Build history of the part. All positions in model axes, mm. A direction names the side the tool comes from. Round coordinates to 2 decimals unless told otherwise and drop trailing zeros. Order: outer loops, then holes, each group sorted by start corner. A loop starts at its lowest first (then second) coordinate and runs counter-clockwise, first axis right, second up. Notation, with made-up numbers: M 10.25,-13.75 L 17.25,-13.75 A27 cw 17.25,24.25 Z; hole C 54.25,-29.5 d9. An arc over 180 degrees is marked long. One line per item, written item: value. Start each with the question number.
Item 1: Tool access for faces 1 (the flat face through (0, 29, -3.099)), 2 (the flat face through (0, 0, 0)), 3 (the flat face through (0, 23.065, -4)): list every direction of +Z, -Z, +X, -X, +Y, -Y with a clear straight run to the whole face (end or side of a thin tool).
Item 2: Probe L1, parallel to Y at x = 4, z = -10; L2, parallel to Y at x = 1, z = -5.25 (3 decimals); L3, parallel to Z at x = -3.5, y = 24.5. List the from-to ranges inside material, lowest first.
Item 3: Band-saw the part on A-A, the plane z = 0. Write the cut outline in (x, y) (1 decimal).
Item 4: Band-saw the part on B-B, the plane x = 0. Write the cut outline in (y, z) (1 decimal), then the cut area to 3 significant figures.
Item 5: Band-saw the part on C-C, the plane y = 5.5. Write the cut outline in (x, z) (1 decimal).
Item 6: Band-saw the part on D-D, the plane y = 21.5. Write the cut outline in (x, z).
Item 7: Pin check, flat tips, straight feed: pin 1 (1 mm diameter, centred on y = 5.5, z = 8, fed in from +X); pin 2 (2 mm diameter, centred on x = 1, z = 4.5, fed in from -Y); pin 3 (5 mm diameter, centred on x = 6.5, y = 9, fed in from -Z); pin 4 (8 mm diameter, centred on y = 11.5, z = 6.5, fed in from +X). Stop position of each tip, or through.
```python
from build123d import *

# Parameters (mm, degrees)
SKETCH1_R           = 11.1125
BOSS_EXTRUDE1_DEPTH = 13.54
SKETCH2_R           = 5.5245
BOSS_EXTRUDE2_DEPTH = 9.525
BOSS_EXTRUDE3_DEPTH = 12.7


with BuildPart() as part:
    # Sketch1 → Boss-Extrude1 (new body)
    with BuildSketch(Plane(origin=(0, 0, 0), x_dir=(1, 0, 0), z_dir=(0, 1, 0))):
        with Locations(Location((0, 0, 0), (0, 0, 270))):
            Circle(SKETCH1_R)
    extrude(amount=BOSS_EXTRUDE1_DEPTH)

    # Sketch2 → Boss-Extrude2 (add)
    with BuildSketch(Plane(origin=(0, 13.54, 0), x_dir=(1, 0, 0), z_dir=(0, 1, 0))):
        with Locations(Location((0, 0, 0), (0, 0, 90))):
            Circle(SKETCH2_R)
    extrude(amount=BOSS_EXTRUDE2_DEPTH)

    # Sketch3 → Boss-Extrude3 (add)
    with BuildSketch(Plane(origin=(0, 23.065, 0), x_dir=(1, 0, 0), z_dir=(0, 1, 0))):
        with BuildLine():
            Line((2.387059513, 3.0988), (-2.387059513, 3.0988))
            ThreePointArc((-2.387059513, 3.0988), (0, -3.9116), (2.387059513, 3.0988))
        make_face()
    extrude(amount=BOSS_EXTRUDE3_DEPTH)


solid = part.part
```
Output:
1. face 1: -Z, +X, -X, +Y
1. face 2: +Z, -Z, +X, -X, -Y
1. face 3: +Y
2. L1: y = 0 to 13.54
2. L2: y = 0 to 23.065
2. L3: z = -1.75 to 1.75
3. outline: M -11.1,0 L 11.1,0 L 11.1,13.5 L 5.5,13.5 L 5.5,23.1 L 3.9,23.1 L 3.9,35.8 L -3.9,35.8 L -3.9,23.1 L -5.5,23.1 L -5.5,13.5 L -11.1,13.5 Z
4. outline: M 0,-11.1 L 13.5,-11.1 L 13.5,-5.5 L 23.1,-5.5 L 23.1,-3.1 L 35.8,-3.1 L 35.8,3.9 L 23.1,3.9 L 23.1,5.5 L 13.5,5.5 L 13.5,11.1 L 0,11.1 Z
4. area: 495 mm²
5. outline: C 0,0 d22.2
6. outline: C 0,0 d11.05
7. pin 1: stops at x = 8.2
7. pin 2: stops at y = 0
7. pin 3: stops at z = -10.37
7. pin 4: stops at x = 10.83
